from build123d import *

# Parameters (mm, degrees)
BOSS_EXTRUDE1_DEPTH   = 6.35
BOSS_EXTRUDE1_2_DEPTH = 6.35


with BuildPart() as part:
    # Sketch1 → Boss-Extrude1 (new body)
    with BuildSketch(Plane(origin=(0, 0, 0), x_dir=(1, 0, 0), z_dir=(0, 1, 0))):
        with BuildLine():
            ThreePointArc((-26.9875, 39.599338196), (-18.852585401, 31.464423597), (-15.875, 20.351923597))
            Line((-15.875, 20.351923597), (-15.875, 0))
            Line((-15.875, 0), (-233.3625, 0))
            Line((-233.3625, 0), (-233.3625, 158.75))
            Line((-233.3625, 158.75), (-26.9875, 39.599338196))
        make_face()
    extrude(amount=BOSS_EXTRUDE1_DEPTH)


with BuildPart() as body_2:
    # Sketch1 → Boss-Extrude1 2 (new body)
    with BuildSketch(Plane(origin=(0, 0, 0), x_dir=(1, 0, 0), z_dir=(0, 1, 0))):
        with BuildLine():
            Line((233.3625, 158.75), (26.9875, 39.599338196))
            ThreePointArc((26.9875, 39.599338196), (18.852585401, 31.464423597), (15.875, 20.351923597))
            Line((15.875, 20.351923597), (15.875, 0))
            Line((15.875, 0), (233.3625, 0))
            Line((233.3625, 0), (233.3625, 158.75))
        make_face()
    extrude(amount=BOSS_EXTRUDE1_2_DEPTH)


solid = body_2.part
Verification items for the finished model (mm, model axes). Coordinates: 2 decimals unless noted, no trailing zeros. Order: outer loops, then holes, each group sorted by start corner. A loop starts at its lowest first (then second) coordinate and runs counter-clockwise, first axis right, second up.
Item 1: Section check C-C, the plane x = 153. Enter the section's corners in (y, z), then the cut area to 3 significant figures.
Filled in:
outline: (0, -112.35) - (6.35, -112.35) - (6.35, 0) - (0, 0) - close
area: 713 mm2
Item 2: Depth check by flat-ended pin: pin 1 (3 mm diameter, centred on x = 110, z = -89.5, fed in from -Y). Enter the tip coordinate at first touch or a pass-through.
Filled in:
pin 1: passes through
Item 3: Section check B-B, the plane z = -74. Enter the section's corners in (x, y), then the cut area to 3 significant figures.
Filled in:
outline: (86.57, 0) - (233.36, 0) - (233.36, 6.35) - (86.57, 6.35) - close
area: 932 mm2
Item 4: Material ranges on L1, parallel to X at y = 2.75, z = -21.5; L2, parallel to Z at x = 59.5, y = 1.5; L3, parallel to X at y = 6.25, z = -90, recorded low to high.
Filled in:
L1: x = 15.9 to 233.36
L2: z = -58.37 to 0
L3: x = 114.28 to 233.36
